Autodesk Inventor part; units mm, degrees
ref_plane "YZ Plane" through (0, 0, 0) normal (1, 0, 0) x (0, 1, 0)
ref_plane "XZ Plane" through (0, 0, 0) normal (0, 1, 0) x (-1, 0, 0)
ref_plane "XY Plane" through (0, 0, 0) normal (0, 0, 1) x (1, 0, 0)
sketch "Sketch1" plane through (0, 0, 0) normal (0, 0, 1) x (1, 0, 0)
  line L0 (90.5, -89.56) -> (-90.5, -89.56)
  line L1 (-90.5, -89.56) -> (-90.5, 89.56)
  line L2 (-90.5, 89.56) -> (90.5, 89.56)
  line L3 (90.5, 89.56) -> (90.5, -89.56)
  line L4 (90.5, -89.56) -> (-90.5, 89.56) construction
  line L5 (-90.5, -89.56) -> (90.5, 89.56) construction
  line L6 (90.5, 89.56) -> (93.65, 89.56)
  line L7 (93.65, 89.56) -> (93.65, 64.56)
  line L8 (93.65, 64.56) -> (90.5, 64.56)
  line L9 (90.5, 64.56) -> (90.5, 89.56)
  line L10 (0, 0) -> (0, 89.56)
  line L11 (-90.5, 89.56) -> (-93.65, 89.56)
  line L12 (-93.65, 89.56) -> (-93.65, 64.56)
  line L13 (-93.65, 64.56) -> (-90.5, 64.56)
  line L14 (-90.5, 64.56) -> (-90.5, 89.56)
  dimension "d0" = 179.12
  dimension "d1" = 181
  dimension "d2" = 3.15
  dimension "d3" = 25
extrude "Extrusion1" add sketch "Sketch1" along normal blind 3.15
sketch "Sketch2" plane through (0, 0, 3.15) normal (0, 0, 1) x (1, 0, 0)
  line L0 (93.65, 89.56) -> (-93.65, 89.56)
  line L1 (-93.65, 89.56) -> (-100.37, 89.56)
  line L2 (-100.37, 89.56) -> (-100.37, 52.06)
  line L3 (-100.37, 52.06) -> (-93.65, 52.06)
  line L4 (-93.65, 52.06) -> (-93.65, 89.56)
  line L5 (0, 89.56) -> (0, 0)
  line L6 (93.65, 89.56) -> (93.65, 64.56)
  line L7 (93.65, 89.56) -> (100.37, 89.56)
  line L8 (100.37, 89.56) -> (100.37, 52.06)
  line L9 (100.37, 52.06) -> (93.65, 52.06)
  line L10 (93.65, 52.06) -> (93.65, 89.56)
  point P0 (-93.65, 64.56)
  dimension "d6" = 6.72
  dimension "d7" = 12.5
extrude "Extrusion2" add sketch "Sketch2" against normal blind 3.15
sketch "Sketch5" plane through (0, 0, 3.15) normal (0, 0, 1) x (1, 0, 0)
  line L0 (-93.65, 64.56) -> (-90.5, 64.56)
  circle A0 centre (-93.65, 64.56) radius 0.25
  circle A1 centre (-90.5, 64.56) radius 0.25
  line L1 (0, 0) -> (0, 89.56)
  line L2 (100.37, 89.56) -> (-100.37, 89.56)
  circle A2 centre (93.65, 64.56) radius 0.25
  circle A3 centre (90.5, 64.56) radius 0.25
  dimension "d19" = 0.5
  dimension "d20" = 0.5
extrude "Extrusion5" cut sketch "Sketch5" against normal up to next
fillet "Fillet1" radius 0.25 2 edges at (-93.65, 52.06, 1.575) (93.65, 52.06, 1.575)
sketch "Sketch3" plane through (-90.5, -89.56, 0) normal (0, -1, 0) x (1, 0, 0)
  line L0 (0, 0) -> (181, 0)
  line L1 (0, 3.15) -> (181, 3.15)
  line L2 (113.65, 3.15) -> (142.85, 3.15)
  line L3 (142.85, 3.15) -> (142.85, 0)
  line L4 (142.85, 0) -> (113.65, 0)
  line L5 (113.65, 0) -> (113.65, 3.15)
  line L6 (128.25, 3.15) -> (128.25, 0)
  point P0 (90.5, 0)
  dimension "d10" = 29.2
  dimension "d11" = 37.75
extrude "Extrusion3" add sketch "Sketch3" along normal blind 20.6
sketch "Sketch4" plane through (0, 0, 3.15) normal (0, 0, 1) x (1, 0, 0)
  line L0 (-90.5, -89.56) -> (23.15, -89.56)
  line L1 (52.35, -110.16) -> (23.15, -110.16)
  circle A0 centre (47.75, -105.16) radius 1.575
  line L2 (0, 0) -> (0, -89.56)
  dimension "d14" = 5
  dimension "d15" = 47.75
  dimension "d16" = 3.15
extrude "Extrusion4" [suppressed]
equation "\"d2\" = t_window"
equation "\"t_door\" = t_window"
equation "\"d8\" = t_door"
equation "\"d12\" = protection_slot_length"
equation "\"d16\" = m3_diameter"
equation "\"wood_thickness\" = 6.72"
equation "\"m3_diameter\" = 3.15"
equation "\"m5_diameter\" = 5.25"
equation "\"stepper_screw_space\" = 35"
equation "\"stepper_shaft_diameter\" = 5"
equation "\"stepper_body_diameter\" = 28"
equation "\"laser_body_diameter\" = 12"
equation "\"thick_acrylic\" = 5.88"
equation "\"carrier_y\" = 181"
equation "\"carrier_z\" = 233.04"
equation "\"carrier_z2\" = 283.04"
equation "\"window_z\" = 185"
equation "\"window_slot\" = 25"
equation "\"reservoir_x\" = 151"
equation "\"reservoir_y\" = 151"
equation "\"thin_acrylic\" = 3.15"
equation "\"linear_bearing_spacing\" = 207"
equation "\"linear_bearing_z\" = 304.8"
equation "\"threaded_rod_z\" = 203.2"
equation "\"motor_spacing\" = 287"
equation "\"tray_boarder\" = 15"
equation "\"tray_x\" = 151"
equation "\"tray_y\" = 181"
equation "\"brass_insert_drill\" = 4"
equation "\"brass_keep_out\" = 8"
equation "\"tape_keep_out\" = 2"
equation "\"tape_thickness\" = 2"
equation "\"crane_x\" = 244.56"
equation "\"z_min_from_center\" = 72.28"
equation "\"printer_z\" = 289"
equation "\"frame_tilt\" = 0"
equation "\"lcd_x\" = 72"
equation "\"lcd_y\" = 25"
equation "\"clear_acrylic\" = 3.15"
equation "\"laser_y\" = 33"
equation "\"laser_y_offset\" = 19.4"
equation "\"laser_diameter\" = 12"
equation "\"laser_z\" = 33"
equation "\"subframe_y_offset\" = 27.5"
equation "\"frame_top_z\" = 295"
equation "\"frame_y\" = 68.44"
equation "\"frame_bottom_z\" = 225"
equation "\"t_frame\" = 6.72"
equation "\"frame_border\" = 39.5"
equation "\"t_carrier\" = 6.72"
equation "\"t_tray\" = 3.15"
equation "\"tray_border\" = 15"
equation "\"t_wall\" = 5.88"
equation "\"galvo_frame_z\" = 65"
equation "\"galvo_frame_x\" = 66"
equation "\"t_galvo_frame\" = 6.72"
equation "\"galvo_frame_y_offset\" = 27.5"
equation "\"m4_diameter\" = 4.2"
equation "\"window_y\" = 49.56"
equation "\"t_window\" = 3.15"
equation "\"laser_x\" = 62"
equation "\"drawer_z\" = 206.72"
equation "\"drawer_x\" = 181"
equation "\"drawer_y\" = 49.56"
equation "\"frame_foot_z\" = 49.5"
equation "\"drawer_z_from_bottom\" = 25"
equation "\"end_stop_offset_x\" = 83"
equation "\"t_crane\" = 6.72"
equation "\"end_stop_spacing\" = 19"
equation "\"thumb_nut_offset_y\" = 11.72"
equation "\"thumb_nut_diameter\" = 7"
equation "\"frame_foot_extension\" = 6"
equation "\"m5_brass_insert_drill\" = 6.7"
equation "\"m3_brass_insert_drill\" = 4"
equation "\"door_sensor\" = 35"
equation "\"protection_slot_offset\" = 37.75"
equation "\"protection_slot\" = 30.2"
equation "\"protection_slot_length\" = 20.6"
equation "\"m3_main_nut_width\" = 5.7"
equation "\"m3_main_extra\" = 1"
equation "\"m3_main_length\" = 14"
equation "\"m3_main_nut_thickness\" = 2.5"
equation "\"al1_thickness\" = 1.5875"
equation "\"bed_t\" = 1.5875"
equation "\"bed_fold_x\" = 15"
equation "\"bed_gap\" = 0.3"
equation "\"bed_y2\" = 45.96"
equation "\"m5_press_nut_drill\" = 6.35"
equation "\"asym_key\" = 0"
equation "\"small_round\" = 2"
equation "\"drawer_foot_mount\" = 18"
equation "\"inner_tray_x\" = 145"
equation "\"t_tape\" = 3"
equation "\"inner_tray_radius\" = 24"
equation "\"t_inner_tray\" = 5.88"
equation "\"inner_tray_border\" = 5"
equation "\"inner_tray_y\" = 145"
equation "\"bottom_clear_border\" = 5"
equation "\"t_bottom_clear\" = 3.15"
equation "\"laser_screw_spacing_y\" = 16"
properties part number "door"
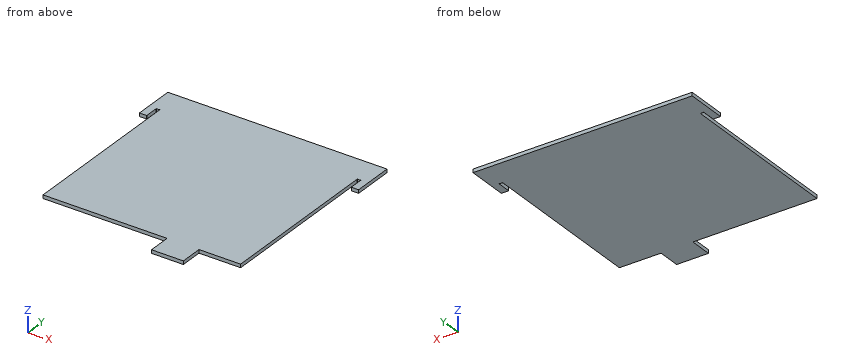
Model file for the job. Use its own axes, mm. Give positions to 0.01 mm unless a question says otherwise; leave off trailing zeros. Order: outer loops, then holes, each group sorted by start corner. A loop starts at its lowest first (then second) coordinate and runs counter-clockwise, first axis right, second up. Notation, with made-up numbers: (-23, -4.75) - (29, -4.75) arc R22 cw to (29, 9.25) - close; hole circle Ø9 at (22.5, 30). An arc over 180 degrees is marked (long way). Return JSON: item names as keys, results as strings.
1) Cut at B-B, the plane y = -85.5. Give the cut face in (x, z), plus the area to 3 significant figures.
Geometry says:
{"outline": "(-90.5, 0) - (90.5, 0) - (90.5, 3.15) - (-90.5, 3.15) - close", "area": "570 mm²"}
2) Cut at C-C, the plane x = 8. Give the cut face in (y, z), plus the area to 3 significant figures.
Geometry says:
{"outline": "(-89.56, 0) - (89.56, 0) - (89.56, 3.15) - (-89.56, 3.15) - close", "area": "564 mm²"}
3) Flat gauge pins, fed straight in: P1, Ø1.6, axis at y = -44.5, z = 1.5, coming from the +X side; P2, Ø1.6, axis at y = 1.5, z = 2, coming from the -X side; P3, Ø0.8, axis at x = -92, z = 2.5, coming from the -Y side. Where does each tip first touch, or does it go through?
Geometry says:
{"P1": "x = 90.5", "P2": "x = -90.5", "P3": "y = 64.56"}
4) Probe line 1 (X direction, y = 54.5, z = 2.65); line 2 (Y direction, x = 19, z = 2.5); line 3 (X direction, y = -52, z = 2.6). List the from-to ranges inside material, lowest first. Write a range as from..to.
Geometry says:
{"line 1": "-100.37..-93.65, -90.5..90.5, 93.65..100.37", "line 2": "-89.56..89.56", "line 3": "-90.5..90.5"}
5) Cut at A-A, the plane z = 1.2. Give the cut face in (x, y), plus the area to 3 significant figures.
Geometry says:
{"outline": "(-100.37, 52.06) - (-93.9, 52.06) arc R0.25 ccw to (-93.65, 52.31) - (-93.65, 64.31) arc R0.25 cw (long way) to (-93.4, 64.56) - (-90.75, 64.56) arc R0.25 cw (long way) to (-90.5, 64.31) - (-90.5, -89.56) - (23.15, -89.56) - (23.15, -110.16) - (52.35, -110.16) - (52.35, -89.56) - (90.5, -89.56) - (90.5, 64.31) arc R0.25 cw (long way) to (90.75, 64.56) - (93.4, 64.56) arc R0.25 cw (long way) to (93.65, 64.31) - (93.65, 52.31) arc R0.25 ccw to (93.9, 52.06) - (100.37, 52.06) - (100.37, 89.56) - (-100.37, 89.56) - close", "area": "33,700 mm²"}
